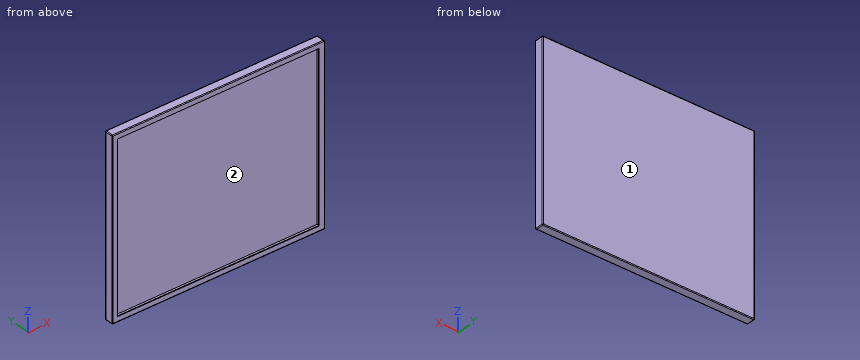
```python
from build123d import *

# Parameters (mm, degrees)
F0_W     = 600
F0_H     = 500
F1_DEPTH = 25
F2_T     = -2
F3_W     = 600
F3_H     = 500
F3_W_2   = 570
F3_H_2   = 470
F4_DEPTH = 2
F5_R     = 2


with BuildPart() as f1:
    # F0 (on Front) → F1 (new body)
    with BuildSketch(Plane.XZ):
        with Locations((0, -50)):
            Rectangle(F0_W, F0_H)
    extrude(amount=-F1_DEPTH)

    # F2
    f2_openings = [f1.faces().sort_by_distance(p)[0] for p in [
        (0, 0, -50),
    ]]
    offset(amount=F2_T, openings=f2_openings)

    # F3 (on Front) → F4 (join)
    with BuildSketch(Plane.XZ):
        with Locations((0, -50)):
            Rectangle(F3_W, F3_H)
        with Locations((0, -50)):
            Rectangle(F3_W_2, F3_H_2, mode=Mode.SUBTRACT)
    extrude(amount=-F4_DEPTH)

    # F5
    f5_edges = [f1.edges().sort_by_distance(p)[0] for p in [
        (-300, 25, -50),
        (0, 25, -300),
        (300, 25, -50),
        (0, 25, 200),
        (-300, 0, -50),
        (0, 0, 200),
        (0, 0, -300),
        (300, 12.5, -300),
        (300, 12.5, 200),
        (-300, 12.5, 200),
        (-300, 12.5, -300),
    ]]
    fillet(f5_edges, radius=F5_R)


solid = f1.part
```
Build history of the part. All positions in model axes, mm. Face numbers are marked on the shaded views. Round coordinates to 2 decimals unless told otherwise and drop trailing zeros. Order: outer loops, then holes, each group sorted by start corner. A loop starts at its lowest first (then second) coordinate and runs counter-clockwise, first axis right, second up. Notation, with made-up numbers: (-11, -23.75) -> (5, -23.75) arc R10 ccw to (5, -4.75) -> close; hole circle Ø4 at (39.25, -19.75). An arc over 180 degrees is marked (long way). Answer in a Markdown table with one row per item.
1) Pin check, flat tips, straight feed: P1, Ø1.6, axis at y = 0.5, z = -61, coming from the -X side; P2, Ø8, axis at x = -79.5, z = 122.5, coming from the -Y side; P3, Ø1.6, axis at x = 111.5, y = 1, coming from the +Z side. Stop position of each tip, or through.
Values:
| item | result |
|---|---|
| P1 | x = -299.87 |
| P2 | y = 23 |
| P3 | z = 199.99 |
2) Band-saw the part on C-C on z = -60. Give the cut face in (x, y).
Values:
| item | result |
|---|---|
| outline | (-300, 2) arc R2 ccw to (-298, 0) -> (-285, 0) -> (-285, 2) -> (-298, 2) -> (-298, 23) -> (298, 23) -> (298, 2) -> (285, 2) -> (285, 0) -> (300, 0) -> (300, 23) arc R2 ccw to (298, 25) -> (-298, 25) arc R2 ccw to (-300, 23) -> close |
3) Band-saw the part on A-A on y = 6.75. Give the cut face in (x, z), and give its area (3 significant figures).
Values:
| item | result |
|---|---|
| outline | (-300, -298) arc R2 ccw to (-298, -300) -> (298, -300) arc R2 ccw to (300, -298) -> (300, 198) arc R2 ccw to (298, 200) -> (-298, 200) arc R2 ccw to (-300, 198) -> close; hole (-298, -298) -> (298, -298) -> (298, 198) -> (-298, 198) -> close |
| area | 4,380 mm2 |
4) Wall check: L1, parallel to Z at x = -219, y = 22.5; L2, parallel to X at y = 22.5, z = 93.5; L3, parallel to X at y = 1.5, z = 90. Give the ranges that are in metal, low to high.
Values:
| item | result |
|---|---|
| L1 | -300 to -298, 198 to 200 |
| L2 | -300 to -298, 298 to 300 |
| L3 | -299.94 to -285, 285 to 300 |
5) Band-saw the part on B-B on x = -53. Give the cut face in (y, z), and give its area (3 significant figures).
Values:
| item | result |
|---|---|
| outline | (0, -298) arc R2 ccw to (2, -300) -> (23, -300) arc R2 ccw to (25, -298) -> (25, 198) arc R2 ccw to (23, 200) -> (2, 200) arc R2 ccw to (0, 198) -> (0, 185) -> (2, 185) -> (2, 198) -> (23, 198) -> (23, -298) -> (2, -298) -> (2, -285) -> (0, -285) -> close |
| area | 1,140 mm2 |
6) Mould opens along X. For the marked faces 1 and 2 say: released by +X, released by -X, zero draft, split by the parting line, or undercut.
Values:
| item | result |
|---|---|
| face 1 | zero draft |
| face 2 | undercut |
